from build123d import *

# Parameters (mm, degrees)
SKETCH1_W           = 30
SKETCH1_H           = 34
BOSS_EXTRUDE1_DEPTH = 3
SKETCH3_W           = 27.5
SKETCH3_H           = 31.5
BOSS_EXTRUDE2_DEPTH = 25.5
FILLET1_R           = 3
BOSS_EXTRUDE3_DEPTH = 5
SKETCH5_OUTSIDE_W   = 42.712
SKETCH5_OUTSIDE_H   = 46.712
SKETCH5_OUTSIDE_W_2 = 5
SKETCH5_OUTSIDE_H_2 = 1
CUT_EXTRUDE1_DEPTH  = 8


with BuildPart() as part:
    # Sketch1 → Boss-Extrude1 (new body)
    with BuildSketch(Plane.XY):
        Rectangle(SKETCH1_W, SKETCH1_H)
    extrude(amount=-BOSS_EXTRUDE1_DEPTH)

    # Sketch3 → Boss-Extrude2 (add)
    with BuildSketch(Plane.XY):
        Rectangle(SKETCH3_W, SKETCH3_H)
    extrude(amount=BOSS_EXTRUDE2_DEPTH)

    # Fillet1
    fillet1_edges = [part.edges().sort_by_distance(p)[0] for p in [
        (13.75, -15.75, 12.75),
        (13.75, 15.75, 12.75),
        (-13.75, 15.75, 12.75),
        (-13.75, -15.75, 12.75),
        (15, -17, -1.5),
        (-15, -17, -1.5),
        (-15, 17, -1.5),
        (15, 17, -1.5),
    ]]
    fillet(fillet1_edges, radius=FILLET1_R)

    # Sketch4 → Boss-Extrude3 (add, symmetric)
    with BuildSketch(Plane(origin=(0, 0, 0), x_dir=(0, 0, -1), z_dir=(1, 0, 0))):
        with BuildLine():
            Line((-2.5, 15.75), (-2.5, 16.5))
            ThreePointArc((-2.5, 16.5), (-2.676424395, 16.881180834), (-3.081195313, 16.993363275))
            Line((-3.081195313, 16.993363275), (-10.636185348, 15.75))
            Line((-10.636185348, 15.75), (-2.5, 15.75))
        make_face()
        with BuildLine():
            Line((-2.5, -15.75), (-10.636185348, -15.75))
            Line((-10.636185348, -15.75), (-3.081195313, -16.993363275))
            ThreePointArc((-3.081195313, -16.993363275), (-2.676424395, -16.881180834), (-2.5, -16.5))
            Line((-2.5, -16.5), (-2.5, -15.75))
        make_face()
    extrude(amount=BOSS_EXTRUDE3_DEPTH, both=True)

    # Sketch5 outside → Cut-Extrude1 (cut)
    with BuildSketch(Plane.XY.offset(25.5)):
        Rectangle(SKETCH5_OUTSIDE_W, SKETCH5_OUTSIDE_H)
        with Locations((-8.597584861, 0)):
            Rectangle(SKETCH5_OUTSIDE_W_2, SKETCH5_OUTSIDE_H_2, mode=Mode.SUBTRACT)
        with Locations((-0.092121408, 12.371641233)):
            Rectangle(SKETCH5_OUTSIDE_W_2, SKETCH5_OUTSIDE_H_2, mode=Mode.SUBTRACT)
        with Locations((-8.993187032, -12.741906988)):
            Rectangle(SKETCH5_OUTSIDE_W_2, SKETCH5_OUTSIDE_H_2, mode=Mode.SUBTRACT)
    extrude(amount=-CUT_EXTRUDE1_DEPTH, mode=Mode.SUBTRACT)


solid = part.part
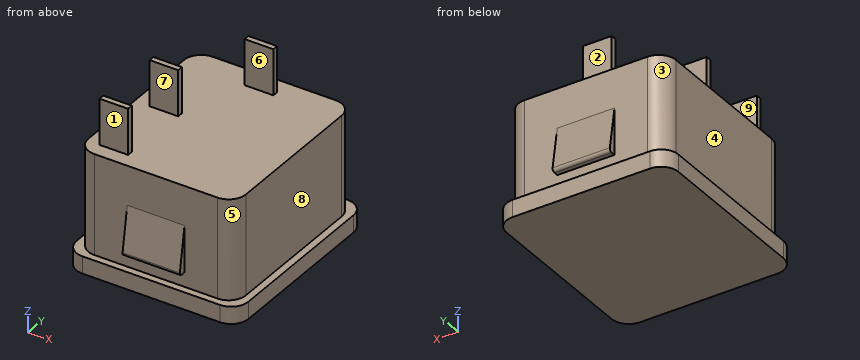
The model under review builds one solid part; all positions refer to its coordinate system, in mm. Face numbers are marked on the shaded views. A direction names the side the tool comes from. Coordinates: 2 decimals unless noted, no trailing zeros. Write each loop counter-clockwise with the first axis right and the second up, starting at its lowest first coordinate (ties: lowest second). Pieces come first, ordered by that corner, then holes. Notation, with made-up numbers: (9, -25.5) - (29, -25.5) arc R31 ccw to (29, 3.5) - close; hole circle Ø6 at (34.25, 1.25). An arc over 180 degrees is marked (long way). Answer as CSV lines item,"result".
(1) Tool access review of the marked faces 1, 2, 3, 4 and 5: name each direction out of +Z, -Z, +X, -X, +Y, -Y from which nothing blocks a thin tool from reaching the whole face with its end or side.
Data:
face 1,"+Z, +X, -X, -Y"
face 2,"+Z, +X, -X, +Y"
face 3,"+Z, -X, +Y"
face 4,"+Z, -X, +Y, -Y"
face 5,"+Z, +X, -Y"
(2) Clearance check with flat-ended pins moving along their axes: pin 1 Ø4 at (x, z) = (-8, 20.5) entering from +Y; pin 2 Ø4 at (x, z) = (-0.5, 20.5) entering from +Y; pin 3 Ø5 at (x, y) = (-10, 9.5) entering from +Z. State where each tip first meets the part, or that it passes through.
Data:
pin 1,"stops at y = 0.5"
pin 2,"stops at y = 12.87"
pin 3,"stops at z = 17.5"
(3) We need section A-A (x = -3.25). Give the boundary of the cut face in (y, z), plus the area to 3 significant figures.
Data:
outline,"(-17, -3) - (17, -3) - (17, 0) - (15.75, 0) - (15.75, 2.5) - (16.5, 2.5) arc R0.5 ccw to (16.99, 3.08) - (15.75, 10.64) - (15.75, 17.5) - (-15.75, 17.5) - (-15.75, 10.64) - (-16.99, 3.08) arc R0.5 ccw to (-16.5, 2.5) - (-15.75, 2.5) - (-15.75, 0) - (-17, 0) - close"
area,"664 mm2"
(4) We need section C-C (z = 13.75). Give the boundary of the cut face in (x, y).
Data:
outline,"(-13.75, -12.75) arc R3 ccw to (-10.75, -15.75) - (10.75, -15.75) arc R3 ccw to (13.75, -12.75) - (13.75, 12.75) arc R3 ccw to (10.75, 15.75) - (-10.75, 15.75) arc R3 ccw to (-13.75, 12.75) - close"
(5) We need section D-D (x = -10). Give the boundary of the cut face in (y, z), plus the area to 3 significant figures.
Data:
outline,"(-17, -3) - (17, -3) - (17, 0) - (15.75, 0) - (15.75, 17.5) - (0.5, 17.5) - (0.5, 25.5) - (-0.5, 25.5) - (-0.5, 17.5) - (-12.24, 17.5) - (-12.24, 25.5) - (-13.24, 25.5) - (-13.24, 17.5) - (-15.75, 17.5) - (-15.75, 0) - (-17, 0) - close"
area,"669 mm2"
(6) Mouldability with a two-part tool opening along Y and no side actions: class the marked faces 6, 7, 8 and 9 as pulls with the +Y half, pulls with the -Y half, needs draft (parallel to the pull), parting line crosses it, or undercut.
Data:
face 6,"pulls with the -Y half"
face 7,"undercut"
face 8,"needs draft"
face 9,"undercut"
(7) For line 1 along Y through (x, z) = (-7.5, 18.25); line 2 along Y through (x, z) = (11, 14.75); line 3 along Z through (x, y) = (10.5, -14), list the stretches that pass through material, from the lowest coordinate up. Write a range as [from, to].
Data:
line 1,"y = [-13.24, -12.24], [-0.5, 0.5]"
line 2,"y = [-15.74, 15.74]"
line 3,"z = [-3, 17.5]"
(8) We need section B-B (y = -8.5). Give the boundary of the cut face in (x, z).
Data:
outline,"(-15, -3) - (15, -3) - (15, 0) - (13.75, 0) - (13.75, 17.5) - (-13.75, 17.5) - (-13.75, 0) - (-15, 0) - close"
